Work out the finished part from the listing and answer in its coordinate system (mm). Coordinates: 2 decimals unless noted, no trailing zeros. Order: outer loops, then holes, each group sorted by start corner. A loop starts at its lowest first (then second) coordinate and runs counter-clockwise, first axis right, second up.
1. The part is cut by section D-D, the plane y = 1.9. Give the vertices of the cut face in (x, z) (3 decimals).
2. Flat-ended cylindrical pins translate along their axes: pin 1 Ø3 at (x, y) = (6, 1.5) entering from +Z; pin 2 Ø3 at (x, y) = (0.5, 3) entering from +Z. Find the tip coordinate at first contact, or state that the pin passes through.
3. The part is cut by section B-B, the plane z = 0. Give the vertices of the cut face in (x, y).
4. Determine the mould class of faces 1 (the cylindrical face through (-11.99, 0.4, -0.53)), 2 (the cylindrical face through (-2.17, 2.96, 9.76)), 3 (the flat face through (-5, 0, -9)) for opening direction X: +X half, -X half, draft (parallel to the pull), parting line (faces both ways), or undercut.
5. Find the intervals of material crossed by probe 1 along X at (y, z) = (3.2, 0); probe 2 along X at (y, z) = (2.8, 4.25); probe 3 along Z at (x, y) = (-8.5, 3.1), in increasing order.
6. The part is cut by section A-A, the plane x = 0. Give the vertices of the cut face in (y, z).
7. The part is cut by section C-C, the plane y = 3.5. Give the vertices of the cut face in (x, z), then the cut area to 3 significant figures.
```python
from build123d import *

# Parameters (mm, degrees)
SKETCH1_R           = 12
SKETCH1_R_2         = 10
BOSS_EXTRUDE1_DEPTH = 6
SKETCH4_R           = 2.5


with BuildPart() as part:
    # Sketch1 → Boss-Extrude1 (new body)
    with BuildSketch(Plane(origin=(0, 0, 0), x_dir=(1, 0, 0), z_dir=(0, 1, 0))):
        Circle(SKETCH1_R)
        Circle(SKETCH1_R_2, mode=Mode.SUBTRACT)
    extrude(amount=BOSS_EXTRUDE1_DEPTH)

    # Sketch4 → Cut-Revolve2 (revolve, cut)
    with BuildSketch(Plane(origin=(0, 0, 0), x_dir=(0, 0, -1), z_dir=(1, 0, 0))):
        with Locations((-13.2, 3)):
            Circle(SKETCH4_R)
    revolve(axis=Axis((0, 0, 0), (0, 1, 0)), mode=Mode.SUBTRACT)


solid = part.part
```
Geometry says:
1. outline: circle Ø21.91 at (0, 0); hole circle Ø20 at (0, 0)
2. pin 1: stops at z = 11.05
2. pin 2: stops at z = 11.19
3. outline: (-12, 0) - (-10, 0) - (-10, 6) - (-12, 6) - (-12, 5.19) arc R2.5 cw to (-12, 0.81) - close; (10, 0) - (12, 0) - (12, 0.81) arc R2.5 cw to (12, 5.19) - (12, 6) - (10, 6) - close
4. face 1: parting line
4. face 2: undercut
4. face 3: draft
5. probe 1: x = -10.71 to -10, 10 to 10.71
5. probe 2: x = -9.83 to -9.05, 9.05 to 9.83
5. probe 3: z = -6.5 to -5.27, 5.27 to 6.5
6. outline: (0, -12) - (0.81, -12) arc R2.5 cw to (5.19, -12) - (6, -12) - (6, -10) - (0, -10) - close; (0, 10) - (6, 10) - (6, 12) - (5.19, 12) arc R2.5 cw to (0.81, 12) - (0, 12) - close
7. outline: circle Ø21.5 at (0, 0); hole circle Ø20 at (0, 0)
7. area: 48.9 mm2
